Check sheet for the modelled part. Datum: model origin and axes. Units: mm. Face numbers are marked on the shaded views. Coordinates: 2 decimals unless noted, no trailing zeros. Order: outer loops, then holes, each group sorted by start corner. A loop starts at its lowest first (then second) coordinate and runs counter-clockwise, first axis right, second up.
1. Draft check along X on the marked faces 1, 2, 3 and 4. Enter one of: released by +X, released by -X, zero draft, split by the parting line, or undercut.
2. Cross-section at C-C (z = 14). Enter the section's corners in (x, y).
3. Gauge pin test, flat ends, axial feed: pin 1 Ø12 at (x, y) = (9.5, 2) entering from -Z (3 decimals); pin 2 Ø2 at (x, z) = (-2, 1.5) entering from -Y; pin 3 Ø1.6 at (x, z) = (58.5, 7.5) entering from -Y. Record the tip position at first contact, or that the pin passes through.
4. Cross-section at A-A (z = 0). Enter the section's corners in (x, y) (1 decimal).
5. Cross-section at D-D (y = 8). Enter the section's corners in (x, z).
6. Thickness scan on line 1 (X direction, y = 1.5, z = 1.5); line 2 (X direction, y = -6.5, z = 16); line 3 (X direction, y = -11, z = -7). Record the ranges inside material, lowest first.
```python
from build123d import *

# Parameters (mm, degrees)
F0_R     = 15.875
F1_DEPTH = 26.9875
F2_R     = 1.5875
F3_DEPTH = 31.75
F4_W     = 1.47257
F4_H     = 21.597792
F5_DEPTH = 19.05


with BuildPart() as f1:
    # F0 (on Right) → F1 (new body, symmetric)
    with BuildSketch(Plane.YZ):
        Circle(F0_R)
    extrude(amount=F1_DEPTH, both=True)

    # F2 (on face) → F3 (join)
    with BuildSketch(Plane.YZ.offset(26.9875)):
        Circle(F2_R)
    extrude(amount=F3_DEPTH)

    # F4 (on Top) → F5 (join, symmetric)
    with BuildSketch(Plane.XY):
        with Locations((58.412209, 0)):
            Rectangle(F4_W, F4_H)
    extrude(amount=F5_DEPTH, both=True)


solid = f1.part
```
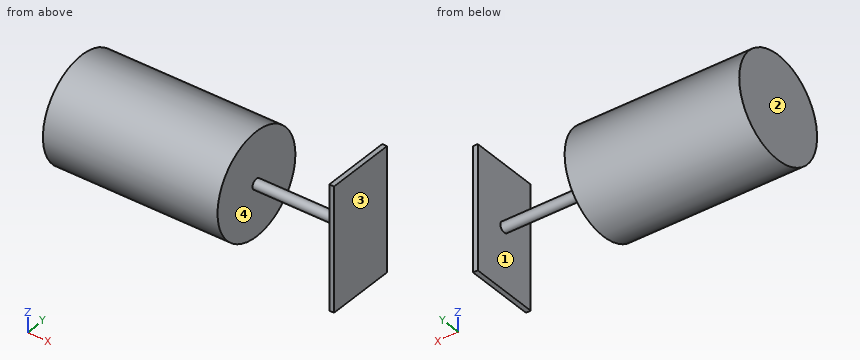
Data:
1. face 1: undercut
1. face 2: released by -X
1. face 3: released by +X
1. face 4: undercut
2. outline: (-26.99, -7.48) - (26.99, -7.48) - (26.99, 7.48) - (-26.99, 7.48) - close; (57.68, -10.8) - (59.15, -10.8) - (59.15, 10.8) - (57.68, 10.8) - close
3. pin 1: stops at z = -15.875
3. pin 2: stops at y = -15.87
3. pin 3: stops at y = -10.8
4. outline: (-27, -15.9) - (27, -15.9) - (27, -1.6) - (57.7, -1.6) - (57.7, -10.8) - (59.1, -10.8) - (59.1, 10.8) - (57.7, 10.8) - (57.7, 1.6) - (27, 1.6) - (27, 15.9) - (-27, 15.9) - close
5. outline: (-26.99, -13.71) - (26.99, -13.71) - (26.99, 13.71) - (-26.99, 13.71) - close; (57.68, -19.05) - (59.15, -19.05) - (59.15, 19.05) - (57.68, 19.05) - close
6. line 1: x = -26.99 to 26.99, 57.68 to 59.15
6. line 2: x = 57.68 to 59.15
6. line 3: x = -26.99 to 26.99
